from build123d import *

# Parameters (mm, degrees)
BOSS_EXTRU_1_DEPTH      = 6.35
ESQUISSE4_R             = 1.778
ENL_V_MAT_EXTRU_2_DEPTH = 7.35
ESQUISSE7_R             = 4.445
ENL_V_MAT_EXTRU_3_DEPTH = 7.35


with BuildPart() as part:
    # Esquisse1 → Boss.-Extru.1 (new body)
    with BuildSketch(Plane(origin=(0, 0, 0), x_dir=(1, 0, 0), z_dir=(0, 1, 0))):
        Polygon((0, 0), (53.975, 0), (53.975, -51.308), (73.025, -51.308), (73.025, -76.454), (53.975, -76.454), (53.975, -114.3), (0, -114.3), align=None)
    boss_extru_1 = extrude(amount=BOSS_EXTRU_1_DEPTH)

    # Symétrie1: Boss.-Extru.1 across plane
    add(boss_extru_1.mirror(Plane(origin=(0, 0, 0), x_dir=(0, 0, 1), z_dir=(1, 0, 0))))

    # Esquisse4 → Enlèv. mat.-Extru.2 (cut, through all)
    with BuildSketch(Plane(origin=(0, 6.35, 0), x_dir=(1, 0, 0), z_dir=(0, 1, 0))):
        with Locations((-50.8, -15.621)):
            Circle(ESQUISSE4_R)
        with Locations((-50.8, -35.179)):
            Circle(ESQUISSE4_R)
        with Locations((50.8, -15.621)):
            Circle(ESQUISSE4_R)
        with Locations((50.8, -35.179)):
            Circle(ESQUISSE4_R)
        with Locations((-4.1, -98.679)):
            Circle(ESQUISSE4_R)
        with Locations((4.1, -98.679)):
            Circle(ESQUISSE4_R)
        with Locations((4.1, -79.121)):
            Circle(ESQUISSE4_R)
        with Locations((-4.1, -79.121)):
            Circle(ESQUISSE4_R)
        with Locations((-50.8, -98.679)):
            Circle(ESQUISSE4_R)
        with Locations((-50.8, -79.121)):
            Circle(ESQUISSE4_R)
        with Locations((50.8, -98.679)):
            Circle(ESQUISSE4_R)
        with Locations((50.8, -79.121)):
            Circle(ESQUISSE4_R)
        with BuildLine():
            Line((-34.17200205, -53.807095184), (-34.17200205, -59.903095184))
            ThreePointArc((-34.17200205, -59.903095184), (-35.95000205, -61.681095184), (-37.72800205, -59.903095184))
            Line((-37.72800205, -59.903095184), (-37.72800205, -53.807095184))
            ThreePointArc((-37.72800205, -53.807095184), (-35.95000205, -52.029095184), (-34.17200205, -53.807095184))
        make_face()
        with BuildLine():
            Line((-17.17199795, -53.807095184), (-17.17199795, -59.903095184))
            ThreePointArc((-17.17199795, -59.903095184), (-18.94999795, -61.681095184), (-20.72799795, -59.903095184))
            Line((-20.72799795, -59.903095184), (-20.72799795, -53.807095184))
            ThreePointArc((-20.72799795, -53.807095184), (-18.94999795, -52.029095184), (-17.17199795, -53.807095184))
        make_face()
        with BuildLine():
            Line((-37.72800205, -67.807092584), (-37.72800205, -73.903092584))
            ThreePointArc((-37.72800205, -73.903092584), (-35.95000205, -75.681092584), (-34.17200205, -73.903092584))
            Line((-34.17200205, -73.903092584), (-34.17200205, -67.807092584))
            ThreePointArc((-34.17200205, -67.807092584), (-35.95000205, -66.029092584), (-37.72800205, -67.807092584))
        make_face()
        with BuildLine():
            Line((-20.72799795, -67.807092584), (-20.72799795, -73.903092584))
            ThreePointArc((-20.72799795, -73.903092584), (-18.94999795, -75.681092584), (-17.17199795, -73.903092584))
            Line((-17.17199795, -73.903092584), (-17.17199795, -67.807092584))
            ThreePointArc((-17.17199795, -67.807092584), (-18.94999795, -66.029092584), (-20.72799795, -67.807092584))
        make_face()
        with BuildLine():
            Line((17.17199795, -67.807092584), (17.17199795, -73.903092584))
            ThreePointArc((17.17199795, -73.903092584), (18.94999795, -75.681092584), (20.72799795, -73.903092584))
            Line((20.72799795, -73.903092584), (20.72799795, -67.807092584))
            ThreePointArc((20.72799795, -67.807092584), (18.94999795, -66.029092584), (17.17199795, -67.807092584))
        make_face()
        with BuildLine():
            Line((20.72799795, -53.807095184), (20.72799795, -59.903095184))
            ThreePointArc((20.72799795, -59.903095184), (18.94999795, -61.681095184), (17.17199795, -59.903095184))
            Line((17.17199795, -59.903095184), (17.17199795, -53.807095184))
            ThreePointArc((17.17199795, -53.807095184), (18.94999795, -52.029095184), (20.72799795, -53.807095184))
        make_face()
        with BuildLine():
            Line((34.17200205, -67.807092584), (34.17200205, -73.903092584))
            ThreePointArc((34.17200205, -73.903092584), (35.95000205, -75.681092584), (37.72800205, -73.903092584))
            Line((37.72800205, -73.903092584), (37.72800205, -67.807092584))
            ThreePointArc((37.72800205, -67.807092584), (35.95000205, -66.029092584), (34.17200205, -67.807092584))
        make_face()
        with BuildLine():
            Line((37.72800205, -53.807095184), (37.72800205, -59.903095184))
            ThreePointArc((37.72800205, -59.903095184), (35.95000205, -61.681095184), (34.17200205, -59.903095184))
            Line((34.17200205, -59.903095184), (34.17200205, -53.807095184))
            ThreePointArc((34.17200205, -53.807095184), (35.95000205, -52.029095184), (37.72800205, -53.807095184))
        make_face()
        with BuildLine():
            Line((-68.08100205, -53.807095184), (-68.08100205, -59.903095184))
            ThreePointArc((-68.08100205, -59.903095184), (-69.85900205, -61.681095184), (-71.63700205, -59.903095184))
            Line((-71.63700205, -59.903095184), (-71.63700205, -53.807095184))
            ThreePointArc((-71.63700205, -53.807095184), (-69.85900205, -52.029095184), (-68.08100205, -53.807095184))
        make_face()
        with BuildLine():
            Line((-71.63700205, -67.807092584), (-71.63700205, -73.903092584))
            ThreePointArc((-71.63700205, -73.903092584), (-69.85900205, -75.681092584), (-68.08100205, -73.903092584))
            Line((-68.08100205, -73.903092584), (-68.08100205, -67.807092584))
            ThreePointArc((-68.08100205, -67.807092584), (-69.85900205, -66.029092584), (-71.63700205, -67.807092584))
        make_face()
        with BuildLine():
            Line((68.08100205, -67.807092584), (68.08100205, -73.903092584))
            ThreePointArc((68.08100205, -73.903092584), (69.85900205, -75.681092584), (71.63700205, -73.903092584))
            Line((71.63700205, -73.903092584), (71.63700205, -67.807092584))
            ThreePointArc((71.63700205, -67.807092584), (69.85900205, -66.029092584), (68.08100205, -67.807092584))
        make_face()
        with BuildLine():
            Line((71.63700205, -53.807095184), (71.63700205, -59.903095184))
            ThreePointArc((71.63700205, -59.903095184), (69.85900205, -61.681095184), (68.08100205, -59.903095184))
            Line((68.08100205, -59.903095184), (68.08100205, -53.807095184))
            ThreePointArc((68.08100205, -53.807095184), (69.85900205, -52.029095184), (71.63700205, -53.807095184))
        make_face()
    extrude(amount=-ENL_V_MAT_EXTRU_2_DEPTH, mode=Mode.SUBTRACT)

    # Esquisse7 → Enlèv. mat.-Extru.3 (cut, through all)
    with BuildSketch(Plane(origin=(0, 6.35, 0), x_dir=(1, 0, 0), z_dir=(0, 1, 0))):
        with Locations((-46.355, -6.35)):
            Circle(ESQUISSE7_R)
        with Locations((46.355, -6.35)):
            Circle(ESQUISSE7_R)
        with Locations((-46.355, -107.95)):
            Circle(ESQUISSE7_R)
        with Locations((46.355, -107.95)):
            Circle(ESQUISSE7_R)
    extrude(amount=-ENL_V_MAT_EXTRU_3_DEPTH, mode=Mode.SUBTRACT)


solid = part.part
Can you work these out from the model? Positions are in its coordinate system, mm. Coordinates: 2 decimals unless noted, no trailing zeros. Write each loop counter-clockwise with the first axis right and the second up, starting at its lowest first coordinate (ties: lowest second). Pieces come first, ordered by that corner, then holes. Notation, with made-up numbers: (19, 53.5) -> (77, 53.5) arc R8 ccw to (77, 61.5) -> close; hole circle Ø8 at (73.25, 72). An arc over 180 degrees is marked (long way). Write each question's results on one line, items separated by ' | '. Start each with the question number.
Q1. Imagine slicing it at A-A (z = 107.95). Write out the boundary of the cut face in (x, y) (3 decimals).
Q2. We'd pull the mould along Z, two halves only. Please class faces 1 (the face through (-52.576, 3.219, 35.101)), 2 (the face through (-53.975, 3, 95)), 3 (the face through (64, 3, 76.454)): +Z half, -Z half, draft (parallel to the pull), parting line (faces both ways), or undercut.
Q3. I'm going to push flat-ended pins straight in: pin 1 (1.5 mm diameter, centred on y = 1, z = 34, fed in from +X) (3 decimals); pin 2 (5.5 mm diameter, centred on x = 50.8, z = 98.679, fed in from +Y). Where does each tip first touch, or does it pass through?
Q4. Imagine slicing it at B-B (x = 4.1). Write out the boundary of the cut face in (y, z).
Q5. Imagine slicing it at C-C (z = 22.5). Write out the boundary of the cut face in (x, y) (3 decimals), then the cut area to 3 significant figures.
Q6. Imagine slicing it at D-D (y = 2.25). State how many separate pieces and enclosed holes the cut face has, then the cut area to 4 significant figures.
Q7. If I drill on probe 1 along X at (y, z) = (3.75, 108) (3 decimals); probe 2 along Z at (x, y) = (-4.1, 4.5); probe 3 along Z at (x, y) = (-51, 2.25), over which ranges is the centre line in solid material (lowest first)?
Taken from the geometry:
1) outline: (-53.975, 0) -> (-50.8, 0) -> (-50.8, 6.35) -> (-53.975, 6.35) -> close; (-41.91, 0) -> (41.91, 0) -> (41.91, 6.35) -> (-41.91, 6.35) -> close; (50.8, 0) -> (53.975, 0) -> (53.975, 6.35) -> (50.8, 6.35) -> close
2) face 1: undercut | face 2: draft | face 3: +Z half
3) pin 1: stops at x = 53.975 | pin 2: stops at y = 6.35
4) outline: (0, 0) -> (6.35, 0) -> (6.35, 77.34) -> (0, 77.34) -> close; (0, 80.9) -> (6.35, 80.9) -> (6.35, 96.9) -> (0, 96.9) -> close; (0, 100.46) -> (6.35, 100.46) -> (6.35, 114.3) -> (0, 114.3) -> close
5) outline: (-53.975, 0) -> (53.975, 0) -> (53.975, 6.35) -> (-53.975, 6.35) -> close | area: 685 mm^2
6) separate pieces: 1 | enclosed holes: 28 | area: 12,550 mm^2
7) probe 1: x = -53.975 to -50.8, -41.91 to 41.91, 50.8 to 53.975 | probe 2: z = 0 to 77.34, 80.9 to 96.9, 100.46 to 114.3 | probe 3: z = 0 to 13.85, 17.39 to 33.41, 36.95 to 77.35, 80.89 to 96.91, 100.45 to 114.3
